Read the model definition and answer for the solid it produces. Units are mm, in the model's axes. Coordinates: 2 decimals unless noted, no trailing zeros. Loops run counter-clockwise (first coordinate to the right, second up) from the corner with the lowest first, then second, coordinate; pieces in that order, holes last. Notation, with made-up numbers: (54, 7) -> (66, 7) arc R31 ccw to (66, 45) -> close; hole circle Ø1 at (-6.75, 16.25). An arc over 180 degrees is marked (long way). Answer as a JSON object with one key per item and string values. Group by question number.
1) Determine the mould class of faces 1 (the face through (-1, -177.8, -25)), 2 (the face through (1, 12.7, -25)), 3 (the face through (1, 0, -17)), 4 (the face through (44, -84, 0)) for opening direction Y: released by +Y, released by -Y, zero draft, split by the parting line, or undercut.
2) Section D-D, the plane z = -24 is taken. Give the vertices of the cut face in (x, y).
3) Consider probe 1 along Y at (x, z) = (32.5, -24); probe 2 along Y at (x, z) = (-12, -9); probe 3 along X at (y, z) = (3.5, -28). Determine where each line is inside the solid, lowest interval first. Write a range as [from, to].
4) Section C-C, the plane x = 17 is taken. Give the vertices of the cut face in (y, z).
5) Section A-A, the plane z = -33.5 is taken. Give the vertices of the cut face in (x, y), plus the area to 3 significant figures.
6) Flat-ended cylindrical pins translate along their axes: P1, Ø10, axis at y = 8.5, z = -34.5, coming from the -X side; P2, Ø1.5, axis at y = -88, z = -38.5, coming from the +X side; P3, Ø10, axis at x = -17.5, y = -64, coming from the +Z side. Find the tip coordinate at first contact, or state that the pin passes through.
7) Section B-B, the plane y = -93.5 is taken. Give the vertices of the cut face in (x, z).
from build123d import *

# Parameters (mm, degrees)
F0_W     = 101.6
F0_H     = 50.8
F1_DEPTH = 177.8
F4_DEPTH = 152.4
F6_DEPTH = 3.81
F8_DEPTH = 12.7


with BuildPart() as f1:
    # F0 (on Front) → F1 (new body)
    with BuildSketch(Plane.XZ):
        with Locations((-0.1263681454, -25.4)):
            Rectangle(F0_W, F0_H)
    extrude(amount=F1_DEPTH)

    # F3 (on Front) → F4 (cut)
    with BuildSketch(Plane.XZ):
        with BuildLine():
            Line((0, -38.1), (0, 0))
            Line((0, 0), (-38.1, 0))
            ThreePointArc((-38.1, 0), (-26.9407683632, -26.9407683632), (0, -38.1))
        make_face()
        with BuildLine():
            Line((38.1, 0), (0, 0))
            Line((0, 0), (0, -38.1))
            ThreePointArc((0, -38.1), (26.9407683632, -26.9407683632), (38.1, 0))
        make_face()
    extrude(amount=F4_DEPTH, mode=Mode.SUBTRACT)

    # F5 (on face) → F6 (cut)
    with BuildSketch(Plane(origin=(0, 0, 0), x_dir=(-1, 0, 0), z_dir=(0, 1, 0))):
        with BuildLine():
            Line((0, -38.1), (0, -44.45))
            ThreePointArc((0, -44.45), (31.4308964237, -31.4308964237), (44.45, 0))
            Line((44.45, 0), (38.1, 0))
            ThreePointArc((38.1, 0), (26.9407683632, -26.9407683632), (0, -38.1))
        make_face()
        with BuildLine():
            Line((-38.1, 0), (-44.45, 0))
            ThreePointArc((-44.45, 0), (-31.4308964237, -31.4308964237), (0, -44.45))
            Line((0, -44.45), (0, -38.1))
            ThreePointArc((0, -38.1), (-26.9407683632, -26.9407683632), (-38.1, 0))
        make_face()
    extrude(amount=-F6_DEPTH, mode=Mode.SUBTRACT)

    # F7 (on face) → F8 (join)
    with BuildSketch(Plane(origin=(0, 0, 0), x_dir=(-1, 0, 0), z_dir=(0, 1, 0))):
        Polygon((50.8, 0), (0, 0), (-50.8, 0), (-50.8, -50.8), (50.8, -50.8), align=None)
    extrude(amount=F8_DEPTH)


solid = f1.part
Determined:
{
 "1": {"face 1": "released by -Y", "face 2": "released by +Y", "face 3": "undercut", "face 4": "zero draft"},
 "2": {"outline": "(-50.93, -177.8) -> (50.67, -177.8) -> (50.67, 0) -> (50.8, 0) -> (50.8, 12.7) -> (-50.8, 12.7) -> (-50.8, 0) -> (-50.93, 0) -> close; hole (-37.41, -3.81) -> (-29.59, -3.81) -> (-29.59, -152.4) -> (29.59, -152.4) -> (29.59, -3.81) -> (37.41, -3.81) -> (37.41, 0) -> (-37.41, 0) -> close"},
 "3": {"probe 1": "[-177.8, -3.81], [0, 12.7]", "probe 2": "[-177.8, -152.4], [0, 12.7]", "probe 3": "[-50.8, 50.8]"},
 "4": {"outline": "(-177.8, -50.8) -> (12.7, -50.8) -> (12.7, 0) -> (0, 0) -> (0, -41.07) -> (-3.81, -41.07) -> (-3.81, -34.1) -> (-152.4, -34.1) -> (-152.4, 0) -> (-177.8, 0) -> close"},
 "5": {"outline": "(-50.93, -177.8) -> (50.67, -177.8) -> (50.67, 0) -> (50.8, 0) -> (50.8, 12.7) -> (-50.8, 12.7) -> (-50.8, 0) -> (-50.93, 0) -> close; hole (-29.22, -3.81) -> (-18.15, -3.81) -> (-18.15, -152.4) -> (18.15, -152.4) -> (18.15, -3.81) -> (29.22, -3.81) -> (29.22, 0) -> (-29.22, 0) -> close", "area": "13,700 mm²"},
 "6": {"P1": "x = -50.8", "P2": "x = 50.67", "P3": "z = -30.75"},
 "7": {"outline": "(-50.93, -50.8) -> (50.67, -50.8) -> (50.67, 0) -> (38.1, 0) arc R38.1 cw to (-38.1, 0) -> (-50.93, 0) -> close"}
}
